from build123d import *
from OCP.BRepFilletAPI import BRepFilletAPI_MakeChamfer

# Parameters (mm, degrees)
SKETCH1_W           = 92
SKETCH1_H           = 67
SKETCH1_W_2         = 88
SKETCH1_H_2         = 57
BOSS_EXTRUDE1_DEPTH = 25
SKETCH2_W           = 92
SKETCH2_H           = 67
BOSS_EXTRUDE2_DEPTH = 0.8
CUT_EXTRUDE1_REACH  = 103.051
SKETCH3_W           = 11
SKETCH3_H           = 7
CUT_EXTRUDE2_DEPTH  = 8
CHAMFER1_SIZE       = 3
CHAMFER1_SIZE2      = 2
CHAMFER2_SIZE       = 2
CHAMFER2_SIZE2      = 3
BOSS_EXTRUDE3_START = 0.8
SKETCH6_R           = 1.6
SKETCH6_W           = 88
SKETCH6_H           = 57
SKETCH6_R_2         = 3.75
SKETCH6_W_2         = 27
SKETCH6_H_2         = 15
BOSS_EXTRUDE3_DEPTH = 0.8
CUT_EXTRUDE3_DEPTH  = 20.8


with BuildPart() as part:
    # Sketch1 → Boss-Extrude1 (new body)
    with BuildSketch(Plane(origin=(0, 0, 0), x_dir=(1, 0, 0), z_dir=(0, 1, 0))):
        Rectangle(SKETCH1_W, SKETCH1_H)
        Rectangle(SKETCH1_W_2, SKETCH1_H_2, mode=Mode.SUBTRACT)
    extrude(amount=BOSS_EXTRUDE1_DEPTH)

    # Sketch2 → Boss-Extrude2 (add)
    with BuildSketch(Plane.XZ):
        Rectangle(SKETCH2_W, SKETCH2_H)
    extrude(amount=BOSS_EXTRUDE2_DEPTH)

    # Sketch3 → Cut-Extrude1 (cut, up to next)
    with BuildSketch(Plane.ZY.offset(46), mode=Mode.PRIVATE) as cut_extrude1_sk1:
        with Locations((0, 15)):
            Rectangle(SKETCH3_W, SKETCH3_H)
    cut_extrude1_tool1 = extrude(cut_extrude1_sk1.sketch, amount=-CUT_EXTRUDE1_REACH, mode=Mode.PRIVATE) & part.part
    add(cut_extrude1_tool1.solids().sort_by_distance((-46, 15, 0))[0], mode=Mode.SUBTRACT)

    # Sketch4 → Cut-Extrude2 (cut)
    with BuildSketch(Plane(origin=(0, 25, 0), x_dir=(1, 0, 0), z_dir=(0, 1, 0))):
        with BuildLine():
            ThreePointArc((-38.4, 31), (-41.13137085, 32.13137085), (-40, 29.4))
            Line((-40, 29.4), (-40, 31))
            Line((-40, 31), (-38.4, 31))
        make_face()
        with BuildLine():
            Line((-40, 31), (-40, 29.4))
            ThreePointArc((-40, 29.4), (-38.86862915, 29.86862915), (-38.4, 31))
            Line((-38.4, 31), (-40, 31))
        make_face()
        with BuildLine():
            ThreePointArc((-40, -29.4), (-41.13137085, -32.13137085), (-38.4, -31))
            Line((-38.4, -31), (-40, -31))
            Line((-40, -31), (-40, -29.4))
        make_face()
        with BuildLine():
            Line((-40, -31), (-38.4, -31))
            ThreePointArc((-38.4, -31), (-38.86862915, -29.86862915), (-40, -29.4))
            Line((-40, -29.4), (-40, -31))
        make_face()
        with BuildLine():
            ThreePointArc((40, -29.4), (38.86862915, -29.86862915), (38.4, -31))
            Line((38.4, -31), (40, -31))
            Line((40, -31), (40, -29.4))
        make_face()
        with BuildLine():
            Line((40, -31), (38.4, -31))
            ThreePointArc((38.4, -31), (40, -32.6), (41.6, -31))
            ThreePointArc((41.6, -31), (41.13137085, -29.86862915), (40, -29.4))
            Line((40, -29.4), (40, -31))
        make_face()
        with BuildLine():
            ThreePointArc((38.4, 31), (38.86862915, 29.86862915), (40, 29.4))
            Line((40, 29.4), (40, 31))
            Line((40, 31), (38.4, 31))
        make_face()
        with BuildLine():
            Line((40, 31), (40, 29.4))
            ThreePointArc((40, 29.4), (41.13137085, 29.86862915), (41.6, 31))
            ThreePointArc((41.6, 31), (40, 32.6), (38.4, 31))
            Line((38.4, 31), (40, 31))
        make_face()
    extrude(amount=-CUT_EXTRUDE2_DEPTH, mode=Mode.SUBTRACT)

    # Chamfer1: one chamfer whose edges measure the first distance from different faces: ONE call of the kernel's chamfer builder (chamfer() names one face for all edges)
    chamfer1_edges_1 = [part.edges().sort_by_distance(p)[0] for p in [
        (46, 12.1, -33.5),
    ]]
    chamfer1_side_1 = [part.faces().sort_by_distance(p)[0] for p in [
        (46, 12.1, 0),
    ]]
    chamfer1_edges_2 = [part.edges().sort_by_distance(p)[0] for p in [
        (-46, 12.1, 33.5),
    ]]
    chamfer1_side_2 = [part.faces().sort_by_distance(p)[0] for p in [
        (-46, 12.1, 32.782041784),
    ]]
    chamfer1 = BRepFilletAPI_MakeChamfer(part.part.solid().wrapped)
    for e in chamfer1_edges_1:
        chamfer1.Add(CHAMFER1_SIZE, CHAMFER1_SIZE2, e.wrapped, chamfer1_side_1[0].wrapped)  # the first distance lies on this face
    for e in chamfer1_edges_2:
        chamfer1.Add(CHAMFER1_SIZE, CHAMFER1_SIZE2, e.wrapped, chamfer1_side_2[0].wrapped)  # the first distance lies on this face
    add(Compound.cast(chamfer1.Shape()), mode=Mode.REPLACE)

    # Chamfer2: one chamfer whose edges measure the first distance from different faces: ONE call of the kernel's chamfer builder (chamfer() names one face for all edges)
    chamfer2_edges_1 = [part.edges().sort_by_distance(p)[0] for p in [
        (-46, 12.1, -33.5),
    ]]
    chamfer2_side_1 = [part.faces().sort_by_distance(p)[0] for p in [
        (-1, 12.1, -33.5),
    ]]
    chamfer2_edges_2 = [part.edges().sort_by_distance(p)[0] for p in [
        (46, 12.1, 33.5),
    ]]
    chamfer2_side_2 = [part.faces().sort_by_distance(p)[0] for p in [
        (1, 12.1, 33.5),
    ]]
    chamfer2 = BRepFilletAPI_MakeChamfer(part.part.solid().wrapped)
    for e in chamfer2_edges_1:
        chamfer2.Add(CHAMFER2_SIZE, CHAMFER2_SIZE2, e.wrapped, chamfer2_side_1[0].wrapped)  # the first distance lies on this face
    for e in chamfer2_edges_2:
        chamfer2.Add(CHAMFER2_SIZE, CHAMFER2_SIZE2, e.wrapped, chamfer2_side_2[0].wrapped)  # the first distance lies on this face
    add(Compound.cast(chamfer2.Shape()), mode=Mode.REPLACE)

    # Sketch6 → Boss-Extrude3 (add)
    # profile 1 of 2: a face of its own
    with BuildSketch(Plane(origin=(0, 25, 0), x_dir=(1, 0, 0), z_dir=(0, 1, 0)).offset(BOSS_EXTRUDE3_START)):
        Polygon((46, 30.5), (44, 33.5), (-44, 33.5), (-46, 30.5), (-46, -30.5), (-44, -33.5), (44, -33.5), (46, -30.5), align=None)
        with Locations(Location((40, -31, 0), (0, 0, 270))):
            Circle(SKETCH6_R, mode=Mode.SUBTRACT)
        with Locations(Location((-40, 31, 0), (0, 0, 270))):
            Circle(SKETCH6_R, mode=Mode.SUBTRACT)
        with Locations(Location((-40, -31, 0), (0, 0, 270))):
            Circle(SKETCH6_R, mode=Mode.SUBTRACT)
        with Locations(Location((40, 31, 0), (0, 0, 270))):
            Circle(SKETCH6_R, mode=Mode.SUBTRACT)
        Rectangle(SKETCH6_W, SKETCH6_H, mode=Mode.SUBTRACT)
    # profile 2 of 2: a face of its own
    with BuildSketch(Plane(origin=(0, 25, 0), x_dir=(1, 0, 0), z_dir=(0, 1, 0)).offset(BOSS_EXTRUDE3_START)):
        Rectangle(SKETCH6_W, SKETCH6_H)
        with Locations(Location((27.5, 2.5, 0), (0, 0, 270))):
            Circle(SKETCH6_R_2, mode=Mode.SUBTRACT)
        with Locations((-15, -1)):
            Rectangle(SKETCH6_W_2, SKETCH6_H_2, mode=Mode.SUBTRACT)
    extrude(amount=-BOSS_EXTRUDE3_DEPTH)

    # Sketch7 → Cut-Extrude3 (cut)
    with BuildSketch(Plane.XZ.offset(0.8)):
        Polygon((-46, 30.5), (-46, -30.5), (-44, -33.5), (44, -33.5), (46, -30.5), (46, 30.5), (44, 33.5), (-44, 33.5), align=None)
    extrude(amount=-CUT_EXTRUDE3_DEPTH, mode=Mode.SUBTRACT)


solid = part.part
Work out the finished part from the listing and answer in its coordinate system (mm). A direction names the side the tool comes from. Round coordinates to 2 decimals unless told otherwise and drop trailing zeros. Write each loop counter-clockwise with the first axis right and the second up, starting at its lowest first coordinate (ties: lowest second). Pieces come first, ordered by that corner, then holes.
1) A cutting plane is placed at A-A (z = -2.5). Give the vertices of the cut face in (x, y).
2) Given pin 1 Ø2.5 at (x, z) = (-40, -31) entering from -Y; pin 2 Ø6 at (x, z) = (-1.5, 8) entering from -Y, each flat-ended and moving along its own axis, determine where each tip first touches the part or whether it passes through.
3) A cutting plane is placed at D-D (x = 15.5). Give the vertices of the cut face in (y, z).
4) A cutting plane is placed at C-C (y = 21.3). Give the vertices of the cut face in (x, z).
5) The mould has two halves that part along X. Classify faces 1 (the cylindrical face through (25.218, 25.406, -5.476)), 2 (the flat face through (-45, 23, -32)), 3 (the flat face through (1, 23, -33.5)), 4 (the flat face through (45, 23, -32)): pulls with the +X half, pulls with the -X half, needs draft (parallel to the pull), parting line crosses it, or undercut.
6) A tool of negligible diameter and unlimited length cuts with its end or side. For faces 5 (the flat face through (-1, 23, 33.5)), 6 (the flat face through (-1, 25, 0)), from which of +Z, -Z, +X, -X, +Y, -Y can it reach the whole face along a straight path? Write none if from no direction.
7) Straight lines are drawn through the part: line 1 (Z direction, x = 40, y = 23.85); line 2 (X direction, y = 20.5, z = -8.5); line 3 (Z direction, x = -12, y = 25.5). For each, find the intervals that lie inside material, in ascending order.
8) A cutting plane is placed at B-B (x = 27.5). Give the vertices of the cut face in (y, z), plus the area to 3 significant figures.
Completed:
1. outline: (-46, 20) - (-44, 20) - (-44, 25) - (-28.5, 25) - (-28.5, 25.8) - (-46, 25.8) - close; (-1.5, 25) - (23.75, 25) - (23.75, 25.8) - (-1.5, 25.8) - close; (31.25, 25) - (44, 25) - (44, 20) - (46, 20) - (46, 25.8) - (31.25, 25.8) - close
2. pin 1: passes through
2. pin 2: stops at y = 25
3. outline: (20, -33.5) - (25.8, -33.5) - (25.8, 33.5) - (20, 33.5) - (20, 28.5) - (25, 28.5) - (25, -28.5) - (20, -28.5) - close
4. outline: (-46, -30.5) - (-44, -33.5) - (44, -33.5) - (46, -30.5) - (46, 30.5) - (44, 33.5) - (-44, 33.5) - (-46, 30.5) - close; hole (-44, -28.5) - (44, -28.5) - (44, 28.5) - (-44, 28.5) - close; hole circle Ø3.2 at (-40, -31); hole circle Ø3.2 at (-40, 31); hole circle Ø3.2 at (40, -31); hole circle Ø3.2 at (40, 31)
5. face 1: undercut
5. face 2: pulls with the -X half
5. face 3: needs draft
5. face 4: pulls with the +X half
6. face 5: +Z, +X, -X, +Y, -Y
6. face 6: -Y
7. line 1: z = -33.5 to -32.6, -29.4 to -28.5, 28.5 to 29.4, 32.6 to 33.5
7. line 2: x = -46 to -44, 44 to 46
7. line 3: z = -33.5 to -6.5, 8.5 to 33.5
8. outline: (20, -33.5) - (25.8, -33.5) - (25.8, -6.25) - (25, -6.25) - (25, -28.5) - (20, -28.5) - close; (20, 28.5) - (25, 28.5) - (25, 1.25) - (25.8, 1.25) - (25.8, 33.5) - (20, 33.5) - close
8. area: 97.6 mm2
